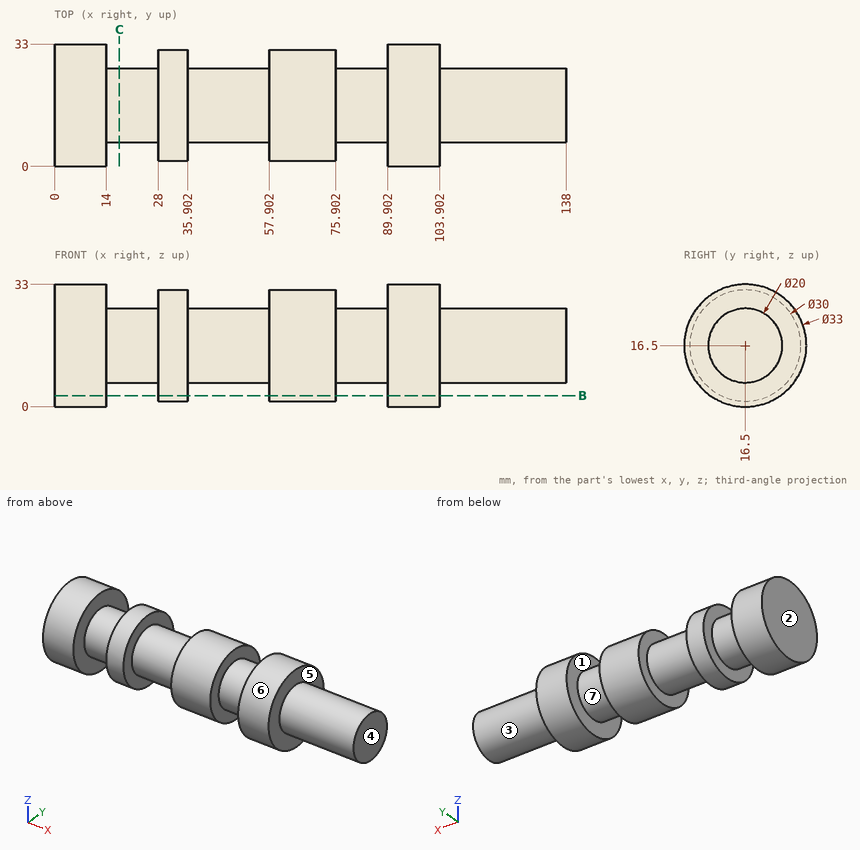
Design review of the part shown in the three views and the two pictorial views. Dimensions are in mm from the part's minimum x, y and z. A direction names the side the tool comes from. Round coordinates to 2 decimals unless told otherwise and drop trailing zeros. Write each loop counter-clockwise with the first axis right and the second up, starting at its lowest first coordinate (ties: lowest second). Pieces come first, ordered by that corner, then holes.
Item 1: We need section B-B on z = 3. Write out the cut boundary in (x, y), and give its area (3 significant figures).
Item 2: For probe 1 along X at (y, z) = (6, 19.5); probe 2 along X at (y, z) = (28, 27); probe 3 along Z at (x, y) = (102.5, 9), list the stretches that pass through material, from the lowest coordinate up.
Item 3: The part is to be moulded in two halves that separate along X. For the marked faces 1, 2, 3 and 4, say which applies: +X half, -X half, draft (parallel to the pull), parting line (faces both ways), or undercut.
Item 4: Clearance check with flat-ended pins moving along their axes: pin 1 Ø1.5 at (x, y) = (27.5, 20) entering from +Z; pin 2 Ø1.5 at (x, z) = (87.5, 24.5) entering from -Y; pin 3 Ø5 at (x, y) = (60, 20) entering from +Z. State where each tip first meets the part, or that it passes through.
Item 5: For the marked faces 5, 6 and 7, list the 3-axis set-ups (+Z, -Z, +X, -X, +Y, -Y) from which the entire face can be reached by the end or side of a thin tool; tool diameter is ignored.
Item 6: We need section C-C on x = 17.5. Write out the cut boundary in (y, z).
Returned:
1. outline: (0, 7.01) - (14, 7.01) - (14, 25.99) - (0, 25.99) - close; (28, 9.96) - (35.9, 9.96) - (35.9, 23.04) - (28, 23.04) - close; (57.9, 9.96) - (75.9, 9.96) - (75.9, 23.04) - (57.9, 23.04) - close; (89.9, 7.01) - (103.9, 7.01) - (103.9, 25.99) - (89.9, 25.99) - close
1. area: 870 mm2
2. probe 1: x = 0 to 14, 28 to 35.9, 57.9 to 75.9, 89.9 to 103.9
2. probe 2: x = 0 to 14, 89.9 to 103.9
2. probe 3: z = 1.8 to 31.2
3. face 1: undercut
3. face 2: -X half
3. face 3: draft
3. face 4: +X half
4. pin 1: stops at z = 31.21
4. pin 2: stops at y = 9.61
4. pin 3: stops at z = 31.47
5. face 5: +X
5. face 6: +X, -X
5. face 7: none
6. outline: circle Ø20 at (16.5, 16.5)
